from build123d import *

# Parameters (mm, degrees)
SKETCH1_W           = 1320
SKETCH1_H           = 788
BOSS_EXTRUDE1_DEPTH = 738
SKETCH5_W           = 1320
SKETCH5_H           = 38
CUT_EXTRUDE1_DEPTH  = 12.7
FILLET2_R           = 2.54
CUT_EXTRUDE2_REACH  = 1067.589
SKETCH6_W           = 38.1
SKETCH6_H           = 788
SKETCH8_W           = 494.5
SKETCH8_H           = 682.6
CUT_EXTRUDE3_DEPTH  = 762.6


with BuildPart() as part:
    # Sketch1 → Boss-Extrude1 (new body)
    with BuildSketch(Plane(origin=(0, 0, 0), x_dir=(1, 0, 0), z_dir=(0, 1, 0))):
        Rectangle(SKETCH1_W, SKETCH1_H)
    extrude(amount=BOSS_EXTRUDE1_DEPTH)

    # Sketch5 → Cut-Extrude1 (cut)
    with BuildSketch(Plane.XY.offset(394)):
        with Locations((0, 689)):
            Rectangle(SKETCH5_W, SKETCH5_H)
    extrude(amount=-CUT_EXTRUDE1_DEPTH, mode=Mode.SUBTRACT)

    # Fillet2
    fillet2_edges = [part.edges().sort_by_distance(p)[0] for p in [
        (0, 708, 394),
        (0, 738, 394),
    ]]
    fillet(fillet2_edges, radius=FILLET2_R)

    # Cut-Extrude2: up to this face of the body (flat: up to its plane)
    cut_extrude2_end = Plane(part.part.faces().sort_by_distance((0, 708, 386.38))[0])
    # Sketch6 → Cut-Extrude2 (cut, up to the picked face)
    with BuildSketch(Plane.XZ, mode=Mode.PRIVATE) as cut_extrude2_sk1:
        with Locations((640.95, 0)):
            Rectangle(SKETCH6_W, SKETCH6_H)
    cut_extrude2_tool1 = split(extrude(cut_extrude2_sk1.sketch, amount=-CUT_EXTRUDE2_REACH, mode=Mode.PRIVATE), bisect_by=cut_extrude2_end, keep=Keep.BOTH, mode=Mode.PRIVATE)
    # Sketch6 → Cut-Extrude2 (cut, up to the picked face)
    with BuildSketch(Plane.XZ, mode=Mode.PRIVATE) as cut_extrude2_sk2:
        with Locations((-640.95, 0)):
            Rectangle(SKETCH6_W, SKETCH6_H)
    cut_extrude2_tool2 = split(extrude(cut_extrude2_sk2.sketch, amount=-CUT_EXTRUDE2_REACH, mode=Mode.PRIVATE), bisect_by=cut_extrude2_end, keep=Keep.BOTH, mode=Mode.PRIVATE)
    add(cut_extrude2_tool1.solids().sort_by(Axis((640.95, 0, 0), (0, 1, 0)))[0], mode=Mode.SUBTRACT)
    add(cut_extrude2_tool2.solids().sort_by(Axis((-640.95, 0, 0), (0, 1, 0)))[0], mode=Mode.SUBTRACT)

    # Sketch8 → Cut-Extrude3 (cut)
    with BuildSketch(Plane.XY.offset(394)):
        with Locations((-349.25, 366.7)):
            Rectangle(SKETCH8_W, SKETCH8_H)
    extrude(amount=-CUT_EXTRUDE3_DEPTH, mode=Mode.SUBTRACT)


solid = part.part
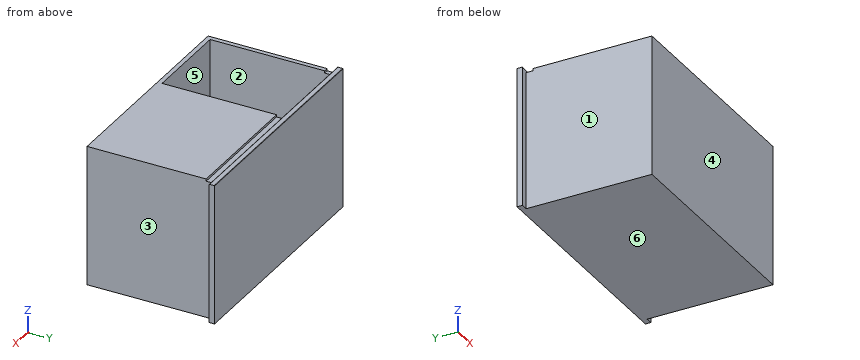
Geometry check sheet. Reference: the model listing, model coordinates, mm. Face numbers are marked on the shaded views. A direction names the side the tool comes from. Round coordinates to 2 decimals unless told otherwise and drop trailing zeros. Write each loop counter-clockwise with the first axis right and the second up, starting at its lowest first coordinate (ties: lowest second). Pieces come first, ordered by that corner, then holes. Notation, with made-up numbers: (3, -40) - (44, -40) arc R18 cw to (44, -27) - close; hole circle Ø11 at (14.25, 57.25). An arc over 180 degrees is marked (long way). One line per item, written item: value.
1. Cross-section at A-A on z = 63.5. Record the boundary of the cut face in (x, y), and give its area (3 significant figures).
The answers:
outline: (-660, 708) - (-621.9, 708) - (-621.9, 0) - (621.9, 0) - (621.9, 708) - (660, 708) - (660, 738) - (-660, 738) - close; hole (-596.5, 25.4) - (-102, 25.4) - (-102, 708) - (-596.5, 708) - close
area: 583,000 mm^2
2. Cross-section at B-B on y = 489. Record the boundary of the cut face in (x, z), and give its area (3 significant figures).
The answers:
outline: (-621.9, -394) - (621.9, -394) - (621.9, 394) - (-102, 394) - (-102, -368.6) - (-596.5, -368.6) - (-596.5, 394) - (-621.9, 394) - close
area: 603,000 mm^2
3. Depth check by flat-ended pin: pin 1 Ø19 at (x, y) = (185.5, 681) entering from +Z; pin 2 Ø10 at (x, y) = (-326.5, 276) entering from +Z; pin 3 Ø10 at (y, z) = (525.5, -216.5) entering from +X. Enter the tip coordinate at first touch or a pass-through.
The answers:
pin 1: stops at z = 381.3
pin 2: stops at z = -368.6
pin 3: stops at x = 621.9
4. Scan lines: L1, parallel to X at y = 226, z = -235; L2, parallel to Y at x = -312, z = 303; L3, parallel to Z at x = -522, y = 363. Record each from-to range of solid material in increasing order.
The answers:
L1: x = -621.9 to -596.5, -102 to 621.9
L2: y = 0 to 25.4, 708 to 738
L3: z = -394 to -368.6
5. Cross-section at C-C on x = -550.5. Record the boundary of the cut face in (y, z).
The answers:
outline: (0, -394) - (738, -394) - (738, 391.46) arc R2.54 ccw to (735.46, 394) - (710.54, 394) arc R2.54 ccw to (708, 391.46) - (708, -368.6) - (25.4, -368.6) - (25.4, 394) - (0, 394) - close
6. Set-up check for the marked faces 1, 2 and 3: record each of +Z, -Z, +X, -X, +Y, -Y from which the full face is reachable in a straight line by a thin tool's end or side.
The answers:
face 1: +Z, -Z, -X, -Y
face 2: +Z
face 3: +Z, -Z, +X, -Y
7. Mould release check, pull along Y, two halves, no side actions. Record for the marked faces 4, 5 and 6: released by +Y, released by -Y, zero draft, split by the parting line, or undercut.
The answers:
face 4: released by -Y
face 5: undercut
face 6: zero draft
